The listing builds one solid part. Answer for the finished solid, in the listing's coordinates (mm). A direction names the side the tool comes from. Give positions to 0.01 mm unless a question says otherwise; leave off trailing zeros. Loops run counter-clockwise (first coordinate to the right, second up) from the corner with the lowest first, then second, coordinate; pieces in that order, holes last. Notation, with made-up numbers: M -9.75,19.5 L 16.25,19.5 A15 ccw 16.25,39.5 Z; hole C 75.25,-11 d4. An arc over 180 degrees is marked long. Return JSON: item names as keys, results as strings.
from build123d import *

# Parameters (mm, degrees)
SKETCH1_W           = 5.9
SKETCH1_H           = 8.2
SKETCH1_W_2         = 8.2
SKETCH1_H_2         = 5.9
BOSS_EXTRUDE1_DEPTH = 8.2
SHELL1_T            = -1.5


with BuildPart() as part:
    # Sketch1 → Boss-Extrude1 (new body)
    with BuildSketch(Plane.XY):
        with Locations((-7.05, 0)):
            Rectangle(SKETCH1_W, SKETCH1_H)
        with Locations((0, 7.05)):
            Rectangle(SKETCH1_W_2, SKETCH1_H_2)
        Rectangle(SKETCH1_W_2, SKETCH1_H)
        with Locations((7.05, 0)):
            Rectangle(SKETCH1_W, SKETCH1_H)
        with Locations((0, -7.05)):
            Rectangle(SKETCH1_W_2, SKETCH1_H_2)
    extrude(amount=BOSS_EXTRUDE1_DEPTH)

    # Shell1
    shell1_openings = [part.faces().sort_by_distance(p)[0] for p in [
        (0, 10, 4.1),
        (10, 0, 4.1),
        (0, -10, 4.1),
        (-10, 0, 4.1),
    ]]
    offset(amount=SHELL1_T, openings=shell1_openings, kind=Kind.INTERSECTION)


solid = part.part
(1) The part is cut by section C-C (y = -5.5). Determine the outline of the cut face in (x, z).
Values follow:
{"outline": "M -4.1,0 L 4.1,0 L 4.1,8.2 L -4.1,8.2 Z; hole M -2.6,1.5 L 2.6,1.5 L 2.6,6.7 L -2.6,6.7 Z"}
(2) Determine the mould class of faces 1 (the flat face through (-2.6, 6, 4)), 2 (the flat face through (-4.1, 7, 4)), 3 (the flat face through (-7, -4.1, 4)) for opening direction X: released by +X, released by -X, zero draft, split by the parting line, or undercut.
Values follow:
{"face 1": "undercut", "face 2": "released by -X", "face 3": "zero draft"}
(3) A tool of negligible diameter and unlimited length cuts with its end or side. For faces 4 (the flat face through (2.6, 6, 4)), 5 (the flat face through (-4.1, -7, 4)), 6 (the flat face through (7, -4.1, 4)), 7 (the flat face through (6, 2.6, 4)), 8 (the flat face through (4.1, 7, 4)), from which of +Z, -Z, +X, -X, +Y, -Y can it reach the whole face along a straight path? Write none if from no direction.
Values follow:
{"face 4": "+Y, -Y", "face 5": "+Z, -Z, -X, -Y", "face 6": "+Z, -Z, +X, -Y", "face 7": "+X, -X", "face 8": "+Z, -Z, +X, +Y"}
(4) The part is cut by section D-D (z = 7.25). Determine the outline of the cut face in (x, y), and give its area (3 significant figures).
Values follow:
{"outline": "M -10,-4.1 L -4.1,-4.1 L -4.1,-10 L 4.1,-10 L 4.1,-4.1 L 10,-4.1 L 10,4.1 L 4.1,4.1 L 4.1,10 L -4.1,10 L -4.1,4.1 L -10,4.1 Z", "area": "261 mm²"}
(5) Straight lines are drawn through the part: line 1 along Z through (x, y) = (-6, 0.75); line 2 along Y through (x, z) = (8.5, 1.75). For each, find the intervals that lie inside material, in ascending order.
Values follow:
{"line 1": "0 to 1.5, 6.7 to 8.2", "line 2": "-4.1 to -2.6, 2.6 to 4.1"}
(6) Given pin 1 (1.6 mm diameter, centred on x = 6.5, z = 5, fed in from +Y); pin 2 (1.8 mm diameter, centred on x = -7.5, z = 5.5, fed in from -Y); pin 3 (2.5 mm diameter, centred on y = -6.5, z = 3, fed in from -X); pin 4 (5 mm diameter, centred on x = 7, y = 7.5, fed in from +Z), each flat-ended and moving along its own axis, determine where each tip first touches the part or whether it passes through.
Values follow:
{"pin 1": "y = 4.1", "pin 2": "y = -4.1", "pin 3": "x = -4.1", "pin 4": "through"}
(7) The part is cut by section A-A (z = 5). Determine the outline of the cut face in (x, y), and give its area (3 significant figures).
Values follow:
{"outline": "M -10,-4.1 L -4.1,-4.1 L -4.1,-10 L -2.6,-10 L -2.6,-2.6 L -10,-2.6 Z; M -10,2.6 L -2.6,2.6 L -2.6,10 L -4.1,10 L -4.1,4.1 L -10,4.1 Z; M 2.6,-10 L 4.1,-10 L 4.1,-4.1 L 10,-4.1 L 10,-2.6 L 2.6,-2.6 Z; M 2.6,2.6 L 10,2.6 L 10,4.1 L 4.1,4.1 L 4.1,10 L 2.6,10 Z", "area": "79.8 mm²"}
(8) The part is cut by section B-B (x = 1.5). Determine the outline of the cut face in (y, z).
Values follow:
{"outline": "M -10,0 L 10,0 L 10,1.5 L -10,1.5 Z; M -10,6.7 L 10,6.7 L 10,8.2 L -10,8.2 Z"}
